Autodesk Inventor part; units mm, degrees
ref_plane "YZ Plane" through (0, 0, 0) normal (1, 0, 0) x (0, 1, 0)
ref_plane "XZ Plane" through (0, 0, 0) normal (0, 1, 0) x (-1, 0, 0)
ref_plane "XY Plane" through (0, 0, 0) normal (0, 0, 1) x (1, 0, 0)
sketch "Szkic1" plane through (0, 0, 0) normal (0, 1, 0) x (-1, 0, 0)
  arc A0 (-4.75, 0) -> (4.75, 0) centre (0, 0) ccw
  line L0 (4.75, 0) -> (-4.75, 0)
  dimension "d0" = 9.5
revolve "Obrót1" add sketch "Szkic1" angle 360 about axis through (-4.75, 0, 0) along (1, 0, 0)
sketch "Szkic2" plane through (0, 0, 0) normal (0, 1, 0) x (-1, 0, 0)
  line L0 (0, 0) -> (0, -26)
  arc A0 (-4.75, -26) -> (4.75, -26) centre (0, -26) ccw
  line L1 (-4.75, -26) -> (4.75, -26)
  dimension "d2" = 26
  dimension "d3" = 9.5
revolve "Obrót2" add sketch "Szkic2" angle 360 about axis through (4.75, 0, -26) along (-1, 0, 0)
sketch "Szkic3" plane through (0, 0, 0) normal (0, 0, 1) x (1, 0, 0)
  circle A0 centre (0, 0) radius 2.5
  dimension "d5" = 5
extrude "Wyciągnięcie proste1" add sketch "Szkic3" against normal blind 26
sketch "Szkic4" plane through (0, 0, 0) normal (1, 0, 0) x (0, 1, 0)
  circle A0 centre (0, 0) radius 2
  circle A1 centre (0, 0) radius 2
  dimension "d8" = 4
  dimension "d11" = 4
extrude "Wyciągnięcie proste2" add sketch "Szkic4" along normal mid plane 17
sketch "Szkic5" plane through (0, 0, 0) normal (0, 1, 0) x (-1, 0, 0)
  line L0 (0, 0) -> (0, -26)
  circle A0 centre (0, -26) radius 2
  dimension "d12" = 26
  dimension "d13" = 4
extrude "Wyciągnięcie proste3" add sketch "Szkic5" along normal mid plane 17
properties part number "wal"
Check sheet for the modelled part. Datum: model origin and axes. Units: mm. A direction names the side the tool comes from. Round coordinates to 2 decimals unless told otherwise and drop trailing zeros. Order: outer loops, then holes, each group sorted by start corner. A loop starts at its lowest first (then second) coordinate and runs counter-clockwise, first axis right, second up.
1) Section check A-A (z = -26). Record the boundary of the cut face in (x, y), and give its area (3 significant figures).
2) Section check B-B (x = 0). Record the boundary of the cut face in (y, z).
3) Go/stop test with flat-tipped pins: pin 1 Ø1.5 at (x, y) = (-1.5, -6) entering from -Z; pin 2 Ø1.5 at (x, y) = (-1, -2.5) entering from -Z; pin 3 Ø10 at (y, z) = (6.5, -20) entering from +X. Record where each tip stops, or that it passes through.
4) Mould release check, pull along Z, two halves, no side actions. Record for faces 1 (the flat face through (0, 8.5, -26)), 2 (the cylindrical face through (-0.54, -2.44, -12.87)): +Z half, -Z half, draft (parallel to the pull), parting line (faces both ways), or undercut.
5) Scan lines: line 1 (Y direction, x = 1.5, z = -13); line 2 (Z direction, x = -2.25, y = 1.5); line 3 (Z direction, x = 1.75, y = -3.25). Record each from-to range of solid material in increasing order.
6) Tool access check on faces 3 (the flat face through (-8.5, 0, 0)), 4 (the cylindrical face through (-6, 0, -2)), 5 (the cylindrical face through (6, 0, 2)), 6 (the cylindrical face through (0, -6, -28)), 7 (the cylindrical face through (-0.923, 6.375, -24.226)). Record the directions out of +Z, -Z, +X, -X, +Y, -Y that give a thin tool (end or side, any length) a straight path to the whole face; none if there is none.
7) Section check C-C (y = -1). Record the boundary of the cut face in (x, z), and give its area (3 significant figures).
8) Section check D-D (y = -6.75). Record the boundary of the cut face in (x, z), and give its area (3 significant figures).
Result:
1. outline: (-2, -8.5) - (2, -8.5) - (2, -4.31) arc R4.75 ccw to (2, 4.31) - (2, 8.5) - (-2, 8.5) - (-2, 4.31) arc R4.75 ccw to (-2, -4.31) - close
1. area: 102 mm2
2. outline: (-8.5, -28) - (-4.31, -28) arc R4.75 ccw to (4.31, -28) - (8.5, -28) - (8.5, -24) - (4.31, -24) arc R4.75 ccw to (2.5, -21.96) - (2.5, -4.04) arc R4.75 ccw (long way) to (-2.5, -4.04) - (-2.5, -21.96) arc R4.75 ccw to (-4.31, -24) - (-8.5, -24) - close
3. pin 1: stops at z = -27.85
3. pin 2: stops at z = -30.33
3. pin 3: stops at x = 2.79
4. face 1: draft
4. face 2: undercut
5. line 1: y = -2 to 2
5. line 2: z = -29.91 to -22.09, -3.91 to 3.91
5. line 3: z = -28.99 to -23.01, -2.99 to 2.99
6. face 3: +Z, -Z, -X, +Y, -Y
6. face 4: -X
6. face 5: +X
6. face 6: -Y
6. face 7: +Y
7. outline: (-8.5, -1.73) - (-4.31, -1.73) arc R4.64 ccw to (-2.29, -4.04) - (-2.29, -21.96) arc R4.64 ccw (long way) to (2.29, -21.96) - (2.29, -4.04) arc R4.64 ccw to (4.31, -1.73) - (8.5, -1.73) - (8.5, 1.73) - (4.31, 1.73) arc R4.64 ccw to (-4.31, 1.73) - (-8.5, 1.73) - close
7. area: 241 mm2
8. outline: circle Ø4 at (0, -26)
8. area: 12.6 mm2
